Part model, mm, in its own coordinate system. A direction names the side the tool comes from. Coordinates: 2 decimals unless noted, no trailing zeros. Write each loop counter-clockwise with the first axis right and the second up, starting at its lowest first coordinate (ties: lowest second). Pieces come first, ordered by that corner, then holes. Notation, with made-up numbers: (-7.5, -7) -> (39.5, -7) arc R11 ccw to (39.5, 6) -> close; hole circle Ø9 at (-13.5, 78.5). An arc over 180 degrees is marked (long way). Write item = value, one per line. Start each with the question number.
Q1. Probe line 1 (Y direction, x = 0, z = 20.7); line 2 (Y direction, x = -5.5, z = 5); line 3 (Z direction, x = 8.25, y = 0.75). List the from-to ranges inside material, lowest first.
Q2. Tool access for faces 4 (the flat face through (9, 0, 0.9)), 5 (the flat face through (4.007, -7.254, 7.27)), 6 (the flat face through (3.5, -6.7, 12.6)), 7 (the flat face through (3.5, -6.7, 5.8)): list every direction of +Z, -Z, +X, -X, +Y, -Y with a clear straight run to the whole face (end or side of a thin tool).
Q3. Band-saw the part on A-A, the plane z = 10.25. List the corners of the cut face in (x, y).
Q4. Pull direction Y, two halves, no side cores. Call faces 1 (the cylindrical face through (-3, 0, 21)), 2 (the flat face through (0, -7.5, 10)), 3 (the flat face through (9, 0, 1.4)): released by +Y, released by -Y, zero draft, split by the parting line, or undercut.
Q5. Pin check, flat tips, straight feed: P1, Ø2, axis at x = 2, y = -1.5, coming from the -Z side; P2, Ø0.6, axis at x = 2.5, y = -7.5, coming from the +Z side; P3, Ø3, axis at y = -5, z = 15, coming from the +X side. Stop position of each tip, or through.
Q6. Band-saw the part on C-C, the plane z = 15. List the corners of the cut face in (x, y), plus the area to 3 significant figures.
from build123d import *

# Parameters (mm, degrees)
SKETCH001_W          = 24
SKETCH001_H          = 24
SKETCH001_W_2        = 22
SKETCH001_H_2        = 15
POCKET_DEPTH         = 20.001
POCKET001_DEPTH      = 18.5
POCKET011_DEPTH      = 1
CHAMFER_SIZE         = 0.98
POCKET009_DEPTH      = 10.001
POCKET009_DEPTH_BACK = 10.001
PAD_DEPTH            = 0.5
POCKET010_DEPTH      = 0.6
PAD001_DEPTH         = 6.8
FILLET001_R          = 0.2
FILLET002_R          = 0.48


with BuildPart() as part:
    # Sketch → Revolution (revolve)
    with BuildSketch(Plane.XZ):
        with BuildLine():
            Line((2.5, 0), (10, 0))
            Line((10, 0), (10, 18.5))
            ThreePointArc((10, 18.5), (9.56066, 19.56066), (8.5, 20))
            Line((8.5, 20), (3, 20))
            Line((3, 20), (3, 21.7))
            Line((3, 21.7), (2.5, 21.7))
            Line((2.5, 21.7), (2.5, 0))
        make_face()
    revolve(axis=Axis((0, 0, 0), (0, 0, 1)))

    # Sketch001 → Pocket (cut, through all)
    with BuildSketch(Plane.XY.offset(20)):
        Rectangle(SKETCH001_W, SKETCH001_H)
        Rectangle(SKETCH001_W_2, SKETCH001_H_2, mode=Mode.SUBTRACT)
    extrude(amount=-POCKET_DEPTH, mode=Mode.SUBTRACT)

    # Sketch002 → Pocket001 (cut)
    with BuildSketch(Plane.XY):
        with BuildLine():
            ThreePointArc((-6.422616, 7), (-9.5, 0), (-6.422616, -7))
            Line((-6.422616, -7), (6.422616, -7))
            ThreePointArc((6.422616, -7), (9.5, 0), (6.422616, 7))
            Line((-6.422616, 7), (6.422616, 7))
        make_face()
    extrude(amount=POCKET001_DEPTH, mode=Mode.SUBTRACT)

    # Sketch016 → Pocket011 (cut)
    with BuildSketch(Plane.XY.offset(18.5)):
        with BuildLine():
            ThreePointArc((-4.821825, 7), (-8.5, 0), (-4.821825, -7))
            Line((-4.821825, -7), (4.821825, -7))
            ThreePointArc((4.821825, -7), (8.5, 0), (4.821825, 7))
            Line((-4.821825, 7), (4.821825, 7))
        make_face()
    extrude(amount=POCKET011_DEPTH, mode=Mode.SUBTRACT)

    # Chamfer
    chamfer_edges = [part.edges().sort_by_distance(p)[0] for p in [
        (8.5, 0, 18.5),
        (-8.5, 0, 18.5),
    ]]
    chamfer(chamfer_edges, length=CHAMFER_SIZE)

    # Sketch011 → Pocket009 (cut, two sides)
    with BuildSketch(Plane.YZ) as pocket009_sk:
        with BuildLine():
            ThreePointArc((-1, 1.4), (-1.5, 1.9), (-2, 1.4))
            Line((-2, 1.4), (-2, -0.5))
            Line((-2, -0.5), (2, -0.5))
            Line((2, 1.4), (2, -0.5))
            ThreePointArc((2, 1.4), (1.5, 1.9), (1, 1.4))
            Line((1, 1.4), (1, 0.9))
            Line((-1, 0.9), (1, 0.9))
            Line((-1, 1.4), (-1, 0.9))
        make_face()
    extrude(amount=-POCKET009_DEPTH, mode=Mode.SUBTRACT)
    extrude(pocket009_sk.sketch, amount=POCKET009_DEPTH_BACK, mode=Mode.SUBTRACT)

    # Sketch012 → Pad (join)
    with BuildSketch(Plane(origin=(0, 0, 1.4), x_dir=(-1, 0, 0), z_dir=(0, 0, -1))):
        with BuildLine():
            Line((9.447222, 1), (8.1, 1))
            Line((8.1, 1), (8.1, -1))
            Line((8.1, -1), (9.447222, -1))
            ThreePointArc((9.447222, -1), (9.5, 0), (9.447222, 1))
        make_face()
        with BuildLine():
            Line((-9.447222, 1), (-8.1, 1))
            Line((-8.1, 1), (-8.1, -1))
            Line((-8.1, -1), (-9.447222, -1))
            ThreePointArc((-9.447222, 1), (-9.5, 0), (-9.447222, -1))
        make_face()
    extrude(amount=PAD_DEPTH)

    # Sketch013 → Pocket010 (cut)
    with BuildSketch(Plane.XZ.offset(7.5)):
        Polygon((2, 12.6), (4.5, 12.6), (4.5, 8.7), (3.5, 5.8), (2, 5.8), align=None)
        Polygon((-4.5, 12.6), (-2, 12.6), (-2, 5.8), (-3.5, 5.8), (-4.5, 8.7), align=None)
    extrude(amount=-POCKET010_DEPTH, mode=Mode.SUBTRACT)

    # Sketch014 → Pad001 (join)
    with BuildSketch(Plane.XY.offset(5.8)):
        with BuildLine():
            Line((2, -7), (4.255262, -6.179152))
            Line((4.255262, -6.179152), (4.426272, -6.648998))
            Line((4.426272, -6.648998), (2.17101, -7.469846))
            ThreePointArc((2, -7.5), (2.086824, -7.492404), (2.17101, -7.469846))
            Line((2, -7), (2, -7.5))
        make_face()
        with BuildLine():
            Line((-2, -7), (-2, -7.5))
            ThreePointArc((-2.17101, -7.469846), (-2.086824, -7.492404), (-2, -7.5))
            Line((-2.17101, -7.469846), (-4.426272, -6.648998))
            Line((-4.426272, -6.648998), (-4.255262, -6.179152))
            Line((-4.255262, -6.179152), (-2, -7))
        make_face()
    extrude(amount=PAD001_DEPTH)

    # Fillet001
    fillet001_edges = [part.edges().sort_by_distance(p)[0] for p in [
        (-6.614378, -7.5, 9.25),
        (-5.626056, -7.5, 19.717894),
        (0, -7.5, 20),
        (5.626056, -7.5, 19.717894),
        (6.614378, -7.5, 9.25),
        (6.614378, 7.5, 9.25),
        (5.626056, 7.5, 19.717894),
        (0, 7.5, 20),
        (-5.626056, 7.5, 19.717894),
        (-6.614378, 7.5, 9.25),
    ]]
    fillet(fillet001_edges, radius=FILLET001_R)

    # Fillet002
    fillet002_edges = [part.edges().sort_by_distance(p)[0] for p in [
        (-10, 0, 0.9),
        (9.987461, 0.500628, 0.9),
        (9.987461, -0.500628, 0.9),
    ]]
    fillet(fillet002_edges, radius=FILLET002_R)


solid = part.part
Ans:
q1.line_1 = -3 to -2.5, 2.5 to 3
q1.line_2 = -7.5 to -7, 7 to 7.5
q1.line_3 = 0.9 to 1.4, 19.5 to 20
q2.face_4 = -Z, +X, -X
q2.face_5 = -Y
q2.face_6 = none
q2.face_7 = -Z
q3.outline = (-6.67, -7.45) arc R0.2 ccw to (-6.54, -7.5) -> (-4.5, -7.5) -> (-4.5, -7) -> (-6.42, -7) arc R9.5 cw to (-6.42, 7) -> (6.42, 7) arc R9.5 cw to (6.42, -7) -> (4.5, -7) -> (4.5, -7.5) -> (6.54, -7.5) arc R0.2 ccw to (6.67, -7.45) arc R10 ccw to (6.67, 7.45) arc R0.2 ccw to (6.54, 7.5) -> (-6.54, 7.5) arc R0.2 ccw to (-6.67, 7.45) arc R10 ccw to start; (-4.43, -6.65) -> (-2.17, -7.47) arc R0.5 ccw to (-2, -7.5) -> (2, -7.5) arc R0.5 ccw to (2.17, -7.47) -> (4.43, -6.65) -> (4.26, -6.18) -> (2, -7) -> (-2, -7) -> (-4.26, -6.18) -> close
q4.face_1 = split by the parting line
q4.face_2 = released by -Y
q4.face_3 = undercut
q5.P1 = 19.5
q5.P2 = 20
q5.P3 = 9.37
q6.outline = (-6.67, -7.45) arc R0.2 ccw to (-6.54, -7.5) -> (6.54, -7.5) arc R0.2 ccw to (6.67, -7.45) arc R10 ccw to (6.67, 7.45) arc R0.2 ccw to (6.54, 7.5) -> (-6.54, 7.5) arc R0.2 ccw to (-6.67, 7.45) arc R10 ccw to start; hole (-6.42, -7) -> (6.42, -7) arc R9.5 ccw to (6.42, 7) -> (-6.42, 7) arc R9.5 ccw to start
q6.area = 29.4 mm2
